Input: part model. Units: mm. Frame: model coordinates. Face numbers are marked on the shaded views. A direction names the side the tool comes from. Coordinates: 2 decimals unless noted, no trailing zeros. Order: outer loops, then holes, each group sorted by start corner. A loop starts at its lowest first (then second) coordinate and runs counter-clockwise, first axis right, second up. Notation, with made-up numbers: M 53.5,70.5 L 98.5,70.5 A30 cw 98.5,103.5 Z; hole C 41,-22.5 d10. An arc over 180 degrees is marked long. One line per item, written item: value.
```python
from build123d import *

# Parameters (mm, degrees)
F0_R          = 16
F1_DEPTH      = 9
F1_DEPTH_BACK = 9
F2_R          = 12
F3_DEPTH      = 7
F3_DEPTH_BACK = 7
F5_DEPTH      = 3
F5_DEPTH_BACK = 3
F7_DEPTH      = 18.001
F8_R          = 5
F9_DEPTH      = 16.001


with BuildPart() as f1:
    # F0 (on Top) → F1 (new body, two sides)
    with BuildSketch(Plane.XY) as f1_sk:
        Circle(F0_R)
    extrude(amount=F1_DEPTH)
    extrude(f1_sk.sketch, amount=-F1_DEPTH_BACK)



with BuildPart() as f3:
    # F2 (on Top) → F3 (new body, two sides)
    with BuildSketch(Plane.XY) as f3_sk:
        with Locations((80, 0)):
            Circle(F2_R)
    extrude(amount=F3_DEPTH)
    extrude(f3_sk.sketch, amount=-F3_DEPTH_BACK)


with BuildPart() as f1_1:
    add(f1.part)

    add(f3.part)  # F5 merges F3
    # F4 (on Top) → F5 (join, two sides)
    with BuildSketch(Plane.XY) as f5_sk:
        Polygon((80.6, 11.9849906133), (0.8, 15.9799874844), (0.8, -15.9799874844), (80.6, -11.9849906133), align=None)
    extrude(amount=F5_DEPTH)
    extrude(f5_sk.sketch, amount=-F5_DEPTH_BACK)

    # F6 (on face) → F7 (cut, through all)
    with BuildSketch(Plane.XY.offset(9)):
        with BuildLine():
            Line((10, 2.5), (6.5383484153, 2.5))
            ThreePointArc((6.5383484153, 2.5), (-7, 0), (6.5383484153, -2.5))
            Line((6.5383484153, -2.5), (10, -2.5))
            ThreePointArc((10, -2.5), (12.5, 0), (10, 2.5))
        make_face()
    extrude(amount=-F7_DEPTH, mode=Mode.SUBTRACT)

    # F8 (on face) → F9 (cut, through all)
    with BuildSketch(Plane.XY.offset(7)):
        with Locations((80, 0)):
            Circle(F8_R)
    extrude(amount=-F9_DEPTH, mode=Mode.SUBTRACT)


solid = f1_1.part
```
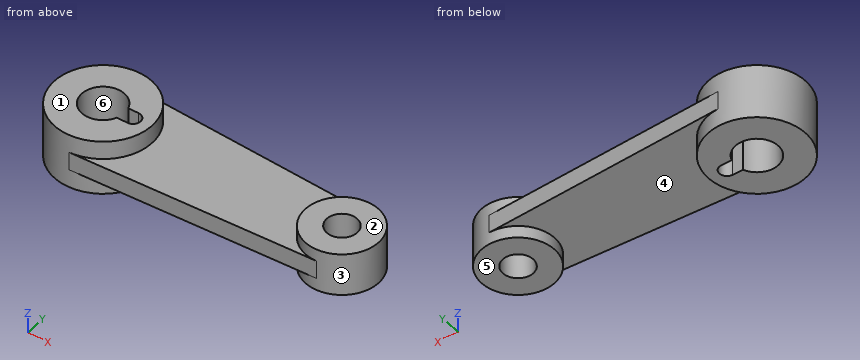
(1) First-contact query: pin 1 (6 mm diameter, centred on y = 11, z = -3.5, fed in from -X); pin 2 (6 mm diameter, centred on x = 77.5, y = 1.5, fed in from +Z); pin 3 (5 mm diameter, centred on x = 36, z = 4.5, fed in from -Y); pin 4 (6 mm diameter, centred on x = 80, y = 0, fed in from -Z). Flat tips, straight axial feed; report the tip coordinate or a pass-through.
Data:
pin 1: stops at x = -13.86
pin 2: stops at z = 7
pin 3: stops at y = -14.32
pin 4: passes through
(2) Access query for the marked faces 1, 2 and 3. Directions: +Z, -Z, +X, -X, +Y, -Y. A direction counts if a zero-diameter tool reaches every point of the face in a straight line with its end or side. Return the directions, or none.
Data:
face 1: +Z, +X, -X, +Y, -Y
face 2: +Z, +X, +Y, -Y
face 3: none
(3) Cut plane A-A on z = -5.5. Output: boundary loops of the cut face in (x, y), plus the area to 3 significant figures.
Data:
outline: C 0,0 d32; C 80,0 d24; hole M 6.54,-2.5 L 10,-2.5 A2.5 ccw 10,2.5 L 6.54,2.5 A7 ccw long Z; hole C 80,0 d10
area: 999 mm2
(4) Cut plane B-B on y = 0. Output: boundary loops of the cut face in (x, z).
Data:
outline: M -16,-9 L -7,-9 L -7,9 L -16,9 Z; M 12.5,-9 L 16,-9 L 16,-3 L 68,-3 L 68,-7 L 75,-7 L 75,7 L 68,7 L 68,3 L 16,3 L 16,9 L 12.5,9 Z; M 85,-7 L 92,-7 L 92,7 L 85,7 Z
(5) Ray query, line 1 (Y direction, x = 80, z = 0); line 2 (Y direction, x = 0, z = 0.75); line 3 (X direction, y = -3, z = -1.5). Return the intervals inside material, ascending. Write a range as from..to.
Data:
line 1: y = -12.02..-5, 5..12.02
line 2: y = -16..-7, 7..16
line 3: x = -15.72..-6.32, 6.32..76, 84..91.62
(6) Cut plane C-C on z = -0.5. Output: boundary loops of the cut face in (x, y) (3 decimals).
Data:
outline: M 0.8,-15.98 L 80.6,-11.985 A12 ccw 80.6,11.985 L 0.8,15.98 A16 ccw long Z; hole M 6.538,-2.5 L 10,-2.5 A2.5 ccw 10,2.5 L 6.538,2.5 A7 ccw long Z; hole C 80,0 d10
(7) Cut plane D-D on x = 37. Output: boundary loops of the cut face in (y, z).
Data:
outline: M -14.17,-3 L 14.17,-3 L 14.17,3 L -14.17,3 Z
(8) Draft query along X for the marked faces 4, 5 and 6. Return one class per face: released by +X, released by -X, zero draft, split by the parting line, or undercut.
Data:
face 4: undercut
face 5: zero draft
face 6: undercut
